Work out the finished part from the listing and answer in its coordinate system (mm). A direction names the side the tool comes from. Coordinates: 2 decimals unless noted, no trailing zeros. Order: outer loops, then holes, each group sorted by start corner. A loop starts at its lowest first (then second) coordinate and runs counter-clockwise, first axis right, second up. Notation, with made-up numbers: M 63,-28.5 L 108,-28.5 A12 cw 108,-22.5 Z; hole C 80.5,17 d10. An arc over 180 degrees is marked long. Write item = value, one per line. Start each with the question number.
Q1. Find section D-D on z = -40.64. Give the vertices of the cut face in (x, y).
Q2. A tool of negligible diameter and unlimited length cuts with its end or side. For faces 4 (the cylindrical face through (-36.488, 40.448, 36.415)), 5 (the flat face through (-33, 0, 1)), 6 (the flat face through (44.45, 40, -1)), 7 (the flat face through (24, 38.1, 1)), 8 (the flat face through (-44.45, 40, -1)), from which of +Z, -Z, +X, -X, +Y, -Y can it reach the whole face along a straight path? Write none if from no direction.
Q3. Determine the mould class of faces 1 (the cylindrical face through (50.25, -2.35, -35.27)), 2 (the flat face through (1, 42.863, 1)), 3 (the flat face through (-2.381, 19, -1)) for opening direction Y: released by +Y, released by -Y, zero draft, split by the parting line, or undercut.
Q4. Find section B-B on y = -1.5. Give the vertices of the cut face in (x, z), and give its area (3 significant figures).
Q5. Each of these flat-tipped pins is pushed along its axis until it touches: P1, Ø8, axis at y = 8.5, z = 13.5, coming from the -X side; P2, Ø7.5, axis at x = 53.34, z = 38.1, coming from the +Y side; P3, Ø1.4, axis at y = 40, z = 15, coming from the -X side; P4, Ø11.5, axis at y = 27, z = 3, coming from the +X side. Where does it stop, or does it pass through?
Q6. Find section A-A on x = -34.29. Give the vertices of the cut face in (y, z).
Q7. Straight lines are drawn through the part: line 1 along Z through (x, y) = (53, -1); line 2 along Z through (x, y) = (34.29, 39.7); line 3 along Y through (x, z) = (-20.5, -19.5). For each, find the intervals that lie inside material, in ascending order.
Q8. Find section C-C on x = -53.34. Give the vertices of the cut face in (y, z).
```python
from build123d import *

# Parameters (mm, degrees)
F0_W     = 127
F0_H     = 101.6
F0_R     = 4.191
F1_DEPTH = 4.7625
F2_W     = 4.7625
F2_H     = 101.6
F3_DEPTH = 38.1
F4_W     = 88.9
F4_H     = 101.6
F4_R     = 4.7625
F5_DEPTH = 4.7625


with BuildPart() as f1:
    # F0 (on Front) → F1 (new body)
    with BuildSketch(Plane.XZ):
        Rectangle(F0_W, F0_H)
        with Locations((-53.34, -38.1)):
            Circle(F0_R, mode=Mode.SUBTRACT)
        with Locations((53.34, -38.1)):
            Circle(F0_R, mode=Mode.SUBTRACT)
        with Locations((-53.34, 38.1)):
            Circle(F0_R, mode=Mode.SUBTRACT)
        with Locations((53.34, 38.1)):
            Circle(F0_R, mode=Mode.SUBTRACT)
    extrude(amount=F1_DEPTH)

    # F2 (on face) → F3 (join)
    with BuildSketch(Plane(origin=(0, 0, 0), x_dir=(-1, 0, 0), z_dir=(0, 1, 0))):
        Rectangle(F2_W, F2_H)
    extrude(amount=F3_DEPTH)

    # F4 (on face) → F5 (join)
    with BuildSketch(Plane(origin=(0, 38.1, 0), x_dir=(-1, 0, 0), z_dir=(0, 1, 0))):
        Rectangle(F4_W, F4_H)
        with Locations((-34.29, -40.64)):
            Circle(F4_R, mode=Mode.SUBTRACT)
        with Locations((34.29, -40.64)):
            Circle(F4_R, mode=Mode.SUBTRACT)
        with Locations((-34.29, 40.64)):
            Circle(F4_R, mode=Mode.SUBTRACT)
        with Locations((34.29, 40.64)):
            Circle(F4_R, mode=Mode.SUBTRACT)
    extrude(amount=F5_DEPTH)


solid = f1.part
```
Findings below:
q1.outline = M -63.5,-4.76 L -56.67,-4.76 L -56.67,0 L -63.5,0 Z; M -50.01,-4.76 L 50.01,-4.76 L 50.01,0 L 2.38,0 L 2.38,38.1 L 29.53,38.1 L 29.53,42.86 L -29.53,42.86 L -29.53,38.1 L -2.38,38.1 L -2.38,0 L -50.01,0 Z; M -44.45,38.1 L -39.05,38.1 L -39.05,42.86 L -44.45,42.86 Z; M 39.05,38.1 L 44.45,38.1 L 44.45,42.86 L 39.05,42.86 Z; M 56.67,-4.76 L 63.5,-4.76 L 63.5,0 L 56.67,0 Z
q2.face_4 = +Y
q2.face_5 = +Z, -Z, -X
q2.face_6 = +Z, -Z, +X, +Y
q2.face_7 = +Z, -Z, +X
q2.face_8 = +Z, -Z, -X, +Y
q3.face_1 = zero draft
q3.face_2 = released by +Y
q3.face_3 = undercut
q4.outline = M -63.5,-50.8 L 63.5,-50.8 L 63.5,50.8 L -63.5,50.8 Z; hole C -53.34,-38.1 d8.38; hole C -53.34,38.1 d8.38; hole C 53.34,-38.1 d8.38; hole C 53.34,38.1 d8.38
q4.area = 12,700 mm^2
q5.P1 = -2.38
q5.P2 = through
q5.P3 = -44.45
q5.P4 = 2.38
q6.outline = M -4.76,-50.8 L 0,-50.8 L 0,50.8 L -4.76,50.8 Z; M 38.1,-50.8 L 42.86,-50.8 L 42.86,-45.4 L 38.1,-45.4 Z; M 38.1,-35.88 L 42.86,-35.88 L 42.86,35.88 L 38.1,35.88 Z; M 38.1,45.4 L 42.86,45.4 L 42.86,50.8 L 38.1,50.8 Z
q7.line_1 = -50.8 to -42.28, -33.92 to 33.92, 42.28 to 50.8
q7.line_2 = -50.8 to -45.4, -35.88 to 35.88, 45.4 to 50.8
q7.line_3 = -4.76 to 0, 38.1 to 42.86
q8.outline = M -4.76,-50.8 L 0,-50.8 L 0,-42.29 L -4.76,-42.29 Z; M -4.76,-33.91 L 0,-33.91 L 0,33.91 L -4.76,33.91 Z; M -4.76,42.29 L 0,42.29 L 0,50.8 L -4.76,50.8 Z
